Design review of the part built by this model. Coordinates are the model's own, in mm. Face numbers are marked on the shaded views. Round coordinates to 2 decimals unless told otherwise and drop trailing zeros. Loops run counter-clockwise (first coordinate to the right, second up) from the corner with the lowest first, then second, coordinate; pieces in that order, holes last. Notation, with made-up numbers: (42.25, 32.25) -> (99.25, 32.25) arc R19 cw to (99.25, 45.25) -> close; hole circle Ø6 at (-6.5, -33). An arc over 180 degrees is marked (long way). Answer as CSV lines item,"result". Start each with the question number.
(1) Take a section at B-B, the plane x = 0. Write out the cut boundary in (y, z).
(2) For P1, Ø5, axis at x = -4, z = 6, coming from the +Y side; P2, Ø1.8, axis at y = 4.5, z = 12, coming from the -X side; P3, Ø1.8, axis at y = 7, z = 11.5, coming from the +X side; P4, Ø5, axis at y = 8, z = 3, coming from the +X side, all flat-tipped, find the tip position at first contact; note any pin that passes through.
(3) Take a section at C-C, the plane y = 8. Write out the cut boundary in (x, z) (3 decimals), and give its area (3 significant figures).
(4) Draft analysis for pull direction X (two halves, no side actions). For the marked faces 1, 2 and 3, state which applies: +X half, -X half, draft (parallel to the pull), parting line (faces both ways), or undercut.
(5) Take a section at A-A, the plane z = 0. Write out the cut boundary in (x, y), and give its area (3 significant figures).
(6) To check wall thickness, follow line 1 (X direction, y = 3.25, z = 0); line 2 (X direction, y = 0.5, z = -2.25); line 3 (Z direction, x = 9.75, y = 9.25). State the ranges of each line that lie inside material, in increasing order. Write a range as from..to.
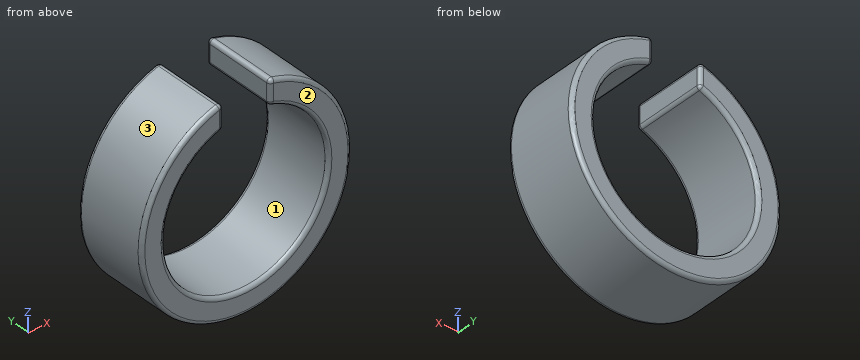
from build123d import *

# Parameters (mm, degrees)
SKETCH1_R           = 14.3
SKETCH1_R_2         = 11.1
BOSS_EXTRUDE1_DEPTH = 10
SKETCH2_W           = 6.35
SKETCH2_H           = 14.3
CUT_EXTRUDE1_DEPTH  = 23.560585099
FILLET1_R           = 0.5


with BuildPart() as part:
    # Sketch1 → Boss-Extrude1 (new body)
    with BuildSketch(Plane(origin=(0, 0, 0), x_dir=(1, 0, 0), z_dir=(0, 1, 0))):
        with Locations(Location((0, 0, 0), (0, 0, 270))):
            Circle(SKETCH1_R)
        with Locations(Location((0, 0, 0), (0, 0, 270))):
            Circle(SKETCH1_R_2, mode=Mode.SUBTRACT)
    extrude(amount=BOSS_EXTRUDE1_DEPTH)

    # Sketch2 → Cut-Extrude1 (cut, through all)
    with BuildSketch(Plane(origin=(0, 0, 0), x_dir=(1, 0, 0), z_dir=(0, 1, 0))):
        with Locations((0, -7.15)):
            Rectangle(SKETCH2_W, SKETCH2_H)
    extrude(amount=CUT_EXTRUDE1_DEPTH, mode=Mode.SUBTRACT)

    # Fillet1
    fillet1_edges = [part.edges().sort_by_distance(p)[0] for p in [
        (3.175, 5, 10.63622936),
        (-3.175, 5, 10.63622936),
        (0, 10, -14.3),
        (0, 0, -14.3),
        (-3.175, 0, 12.289652799),
        (3.175, 0, 12.289652799),
        (3.175, 10, 12.289652799),
        (-3.175, 10, 12.289652799),
        (-3.175, 5, 13.943076239),
        (3.175, 5, 13.943076239),
        (0, 0, -11.1),
        (0, 10, -11.1),
    ]]
    fillet(fillet1_edges, radius=FILLET1_R)


solid = part.part
The answers:
1,outline,"(0, -13.8) arc R0.5 ccw to (0.5, -14.3) -> (9.5, -14.3) arc R0.5 ccw to (10, -13.8) -> (10, -11.6) arc R0.5 ccw to (9.5, -11.1) -> (0.5, -11.1) arc R0.5 ccw to (0, -11.6) -> close"
2,P1,"through"
2,P2,"x = -9.02"
2,P3,"x = 9.6"
2,P4,"x = 14.29"
3,outline,"(-3.808, 13.784) arc R14.3 ccw (long way) to (3.808, 13.784) arc R0.5 ccw to (3.175, 13.302) -> (3.175, 11.002) arc R0.5 ccw to (3.517, 10.528) arc R11.1 cw (long way) to (-3.517, 10.528) arc R0.5 ccw to (-3.175, 11.002) -> (-3.175, 13.302) arc R0.5 ccw to start"
3,area,"235 mm²"
4,face 1,"undercut"
4,face 2,"draft"
4,face 3,"parting line"
5,outline,"(-14.3, 0.5) arc R0.5 ccw to (-13.8, 0) -> (-11.6, 0) arc R0.5 ccw to (-11.1, 0.5) -> (-11.1, 9.5) arc R0.5 ccw to (-11.6, 10) -> (-13.8, 10) arc R0.5 ccw to (-14.3, 9.5) -> close; (11.1, 0.5) arc R0.5 ccw to (11.6, 0) -> (13.8, 0) arc R0.5 ccw to (14.3, 0.5) -> (14.3, 9.5) arc R0.5 ccw to (13.8, 10) -> (11.6, 10) arc R0.5 ccw to (11.1, 9.5) -> close"
5,area,"63.6 mm²"
6,line 1,"-14.3..-11.1, 11.1..14.3"
6,line 2,"-14.12..-10.87, 10.87..14.12"
6,line 3,"-10.46..-5.31, 5.31..10.46"
